from build123d import *

# Parameters (mm, degrees)
F3_DEPTH = 0.3
F4_R     = 1.5
F5_DEPTH = 4.5
F6_R     = 0.5
F8_DEPTH = 0.301


with BuildPart() as f3:
    # F2 (on Top) → F3 (new body)
    with BuildSketch(Plane.XY):
        with BuildLine():
            ThreePointArc((21.9341482237, -0.1564722617), (21.9660226591, 0), (21.9341482237, 0.1564722617))
            ThreePointArc((21.9341482237, 0.1564722617), (0, 14.6666666667), (-21.9341482237, 0.1564722617))
            ThreePointArc((-21.9341482237, 0.1564722617), (-21.9660226591, 0), (-21.9341482237, -0.1564722617))
            ThreePointArc((-21.9341482237, -0.1564722617), (0, -14.6666666667), (21.9341482237, -0.1564722617))
        make_face()
    extrude(amount=F3_DEPTH)

    # F4 (on face) → F5 (join)
    with BuildSketch(Plane.XY.offset(0.3)):
        with Locations((-5, 0)):
            Circle(F4_R)
        with Locations((5, 0)):
            Circle(F4_R)
    extrude(amount=F5_DEPTH)

    # F6
    f6_edges = [f3.edges().sort_by_distance(p)[0] for p in [
        (-6.5, 0, 4.8),
        (3.5, 0, 4.8),
    ]]
    fillet(f6_edges, radius=F6_R)

    # F7 (on face) → F8 (cut, through all)
    with BuildSketch(Plane.XY.offset(0.3)):
        with BuildLine():
            ThreePointArc((-0.3870967742, -12.5971768966), (0, -12.8963994815), (0.3870967742, -12.5971768966))
            ThreePointArc((0.3870967742, -12.5971768966), (2, 0), (0.3870967742, 12.5971768966))
            ThreePointArc((0.3870967742, 12.5971768966), (0, 12.8963994815), (-0.3870967742, 12.5971768966))
            ThreePointArc((-0.3870967742, 12.5971768966), (-2, 0), (-0.3870967742, -12.5971768966))
        make_face()
    extrude(amount=-F8_DEPTH, mode=Mode.SUBTRACT)


solid = f3.part
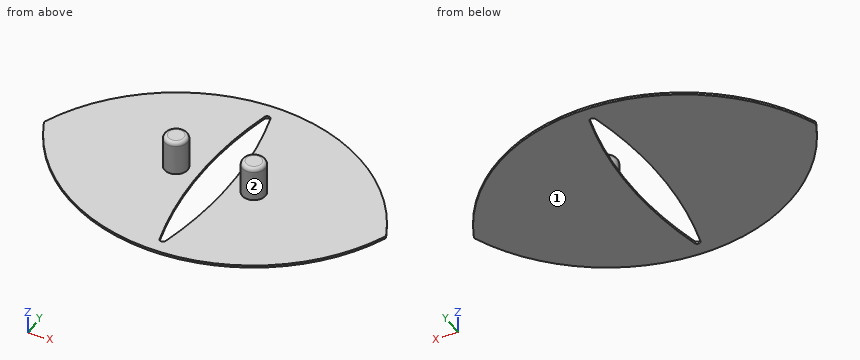
Verification items for the finished model (mm, model axes). Face numbers are marked on the shaded views. Give positions to 0.01 mm unless a question says otherwise; leave off trailing zeros. Write each loop counter-clockwise with the first axis right and the second up, starting at its lowest first coordinate (ties: lowest second). Pieces come first, ordered by that corner, then holes. Notation, with made-up numbers: M 74.25,56 L 102.25,56 A11 cw 102.25,69 Z; hole C 75,71.5 d10. An arc over 180 degrees is marked long. Write item = value, one per line.
(1) Go/stop test with flat-tipped pins: pin 1 Ø3 at (x, y) = (-8, -2) entering from +Z; pin 2 Ø2 at (y, z) = (-6.5, 1) entering from +X. Record where each tip stops, or that it passes through.
Found:
pin_1 = 0.3
pin_2 = 18.56
(2) Draft check along X on the marked faces 1 and 2. Enter one of: released by +X, released by -X, zero draft, split by the parting line, or undercut.
Found:
face_1 = zero draft
face_2 = undercut
(3) Sectioned sample at B-B (z = 3.05). Record the cut outline in (x, y), then the cut area to 3 significant figures.
Found:
outline = C -5,0 d3; C 5,0 d3
area = 14.1 mm2
(4) Material ranges on line 1 (Z direction, x = -8, y = 11.75); line 2 (Y direction, x = 5.5, z = 3.3), recorded low to high.
Found:
line_1 = 0 to 0.3
line_2 = -1.41 to 1.41
(5) Sectioned sample at C-C (x = -5). Record the cut outline in (y, z), then the cut area to 3 significant figures.
Found:
outline = M -14.14,0 L 14.14,0 L 14.14,0.3 L 1.5,0.3 L 1.5,4.3 A0.5 ccw 1,4.8 L -1,4.8 A0.5 ccw -1.5,4.3 L -1.5,0.3 L -14.14,0.3 Z
area = 21.9 mm2
(6) Sectioned sample at D-D (y = -11.5). Record the cut outline in (x, z).
Found:
outline = M -11.87,0 L -0.66,0 L -0.66,0.3 L -11.87,0.3 Z; M 0.66,0 L 11.87,0 L 11.87,0.3 L 0.66,0.3 Z
(7) Sectioned sample at A-A (y = 6). Record the cut outline in (x, z).
Found:
outline = M -18.38,0 L -1.64,0 L -1.64,0.3 L -18.38,0.3 Z; M 1.64,0 L 18.38,0 L 18.38,0.3 L 1.64,0.3 Z
